```python
from build123d import *

# Parameters (mm, degrees)
SKETCH1_W           = 40
SKETCH1_H           = 80
SKETCH1_R           = 4
BOSS_EXTRUDE1_DEPTH = 4
CHAMFER1_SIZE       = 3.5


with BuildPart() as part:
    # Sketch1 → Boss-Extrude1 (new body)
    with BuildSketch(Plane(origin=(0, 0, 0), x_dir=(0, 0, -1), z_dir=(1, 0, 0))):
        with Locations((0, -82.5)):
            Rectangle(SKETCH1_W, SKETCH1_H)
        with Locations((0, -62.5)):
            Circle(SKETCH1_R, mode=Mode.SUBTRACT)
    extrude(amount=BOSS_EXTRUDE1_DEPTH)

    # Chamfer1
    chamfer1_edges = [part.edges().sort_by_distance(p)[0] for p in [
        (0, -62.5, 4),
    ]]
    chamfer(chamfer1_edges, length=CHAMFER1_SIZE)


solid = part.part
```
Build history of the part. All positions in model axes, mm. Round coordinates to 2 decimals unless told otherwise and drop trailing zeros. Write each loop counter-clockwise with the first axis right and the second up, starting at its lowest first coordinate (ties: lowest second). Pieces come first, ordered by that corner, then holes. Notation, with made-up numbers: (-12.5, 79) -> (8.5, 79) arc R23 cw to (8.5, 101) -> close; hole circle Ø11 at (20, -33). An arc over 180 degrees is marked (long way). Put each result on its own line as item: value.
Item 1: Wall check: probe 1 along Y at (x, z) = (3.8, 0); probe 2 along Y at (x, z) = (3.5, -2.5). Give the ranges that are in metal, low to high. Write a range as from..to.
Here are the results:
probe 1: y = -122.5..-66.5, -58.5..-42.5
probe 2: y = -122.5..-65.62, -59.38..-42.5
Item 2: Slice it at A-A, the plane z = 0. Give the cut face in (x, y), plus the area to 3 significant figures.
Here are the results:
outline: (0, -122.5) -> (4, -122.5) -> (4, -66.5) -> (3.5, -66.5) -> (0, -70) -> close; (0, -55) -> (3.5, -58.5) -> (4, -58.5) -> (4, -42.5) -> (0, -42.5) -> close
area: 276 mm^2
Item 3: Flat gauge pin, fed straight in: P1, Ø8, axis at y = -64.5, z = 1, coming from the -X side. Where does the tip first touch, or does it go through?
Here are the results:
P1: stops at x = 1.26
Item 4: Slice it at B-B, the plane y = -62.5. Give the cut face in (x, z).
Here are the results:
outline: (0, -20) -> (4, -20) -> (4, -4) -> (3.5, -4) -> (0, -7.5) -> close; (0, 7.5) -> (3.5, 4) -> (4, 4) -> (4, 20) -> (0, 20) -> close
Item 5: Slice it at C-C, the plane x = 1.15. Give the cut face in (y, z).
Here are the results:
outline: (-122.5, -20) -> (-42.5, -20) -> (-42.5, 20) -> (-122.5, 20) -> close; hole circle Ø12.7 at (-62.5, 0)
Item 6: Two-plate mould, pull along Z, no slides. Class faces 1 (the face through (2, -42.5, 0)), 2 (the face through (3.281, -61.233, -4.024)), 3 (the face through (2, -83, -20)): pulls with the +Z half, pulls with the -Z half, needs draft (parallel to the pull), parting line crosses it, or undercut.
Here are the results:
face 1: needs draft
face 2: undercut
face 3: pulls with the -Z half
